```python
from build123d import *

# Parameters (mm, degrees)
SKETCH013_R     = 3.96875
PAD009_DEPTH    = 164
SKETCH014_R     = 7.5
PAD010_DEPTH    = 10
SKETCH015_R     = 7.5
POCKET003_DEPTH = 8
SKETCH016_R     = 7.5
SKETCH016_R_2   = 3.96875
POCKET004_DEPTH = 2
SKETCH017_R     = 7.5
PAD011_DEPTH    = 10
SKETCH018_R     = 7.5
POCKET005_DEPTH = 8
SKETCH019_R     = 7.5
SKETCH019_R_2   = 3.96875
POCKET006_DEPTH = 2


with BuildPart() as part:
    # Sketch013 → Pad009 (new body)
    with BuildSketch(Plane(origin=(500, 82, 56), x_dir=(1, 0, 0), z_dir=(0, -1, 0))):
        Circle(SKETCH013_R)
    extrude(amount=PAD009_DEPTH)

    # Sketch014 → Pad010 (new body)
    with BuildSketch(Plane(origin=(500, 82, 56), x_dir=(1, 0, 0), z_dir=(0, 1, 0))):
        Circle(SKETCH014_R)
    extrude(amount=-PAD010_DEPTH)

    # Sketch015 → Pocket003 (cut)
    with BuildSketch(Plane(origin=(500, 82, 56), x_dir=(1, 0, 0), z_dir=(0, 1, 0))):
        Circle(SKETCH015_R)
        Polygon((0, 5), (-4.330127, 2.5), (-4.330127, -2.5), (0, -5), (4.330127, -2.5), (4.330127, 2.5), align=None, mode=Mode.SUBTRACT)
    extrude(amount=-POCKET003_DEPTH, mode=Mode.SUBTRACT)

    # Sketch016 → Pocket004 (cut)
    with BuildSketch(Plane(origin=(500, 82, 56), x_dir=(1, 0, 0), z_dir=(0, 1, 0))):
        Circle(SKETCH016_R)
        Circle(SKETCH016_R_2, mode=Mode.SUBTRACT)
    extrude(amount=-POCKET004_DEPTH, mode=Mode.SUBTRACT)

    # Sketch017 → Pad011 (new body)
    with BuildSketch(Plane(origin=(500, -82, 56), x_dir=(1, 0, 0), z_dir=(0, -1, 0))):
        Circle(SKETCH017_R)
    extrude(amount=-PAD011_DEPTH)

    # Sketch018 → Pocket005 (cut)
    with BuildSketch(Plane(origin=(500, -82, 56), x_dir=(1, 0, 0), z_dir=(0, -1, 0))):
        Circle(SKETCH018_R)
        Polygon((0, 5), (-4.330127, 2.5), (-4.330127, -2.5), (0, -5), (4.330127, -2.5), (4.330127, 2.5), align=None, mode=Mode.SUBTRACT)
    extrude(amount=-POCKET005_DEPTH, mode=Mode.SUBTRACT)

    # Sketch019 → Pocket006 (cut)
    with BuildSketch(Plane(origin=(500, -82, 56), x_dir=(1, 0, 0), z_dir=(0, -1, 0))):
        Circle(SKETCH019_R)
        Circle(SKETCH019_R_2, mode=Mode.SUBTRACT)
    extrude(amount=-POCKET006_DEPTH, mode=Mode.SUBTRACT)


with BuildPart() as part_1:
    # Clone020 placement: moved
    add(part.part.moved(Location((-951.5, 0, -84))))


solid = part_1.part
```
Model file for the job. Use its own axes, mm. A direction names the side the tool comes from. Coordinates: 2 decimals unless noted, no trailing zeros. Order: outer loops, then holes, each group sorted by start corner. A loop starts at its lowest first (then second) coordinate and runs counter-clockwise, first axis right, second up. Notation, with made-up numbers: (89.25, -33.75) -> (123.25, -33.75) arc R24 cw to (123.25, -4.75) -> close; hole circle Ø8 at (-40, -26.5). An arc over 180 degrees is marked (long way). Return JSON: item names as keys, results as strings.
Item 1: Wall check: line 1 along Y through (x, z) = (-453.5, -33.5); line 2 along Y through (x, z) = (-447.5, -28.5); line 3 along X through (y, z) = (-49, -25.5). Give the ranges that are in metal, low to high. Write a range as from..to.
Model answer:
{"line 1": "y = -74..-72, 72..74", "line 2": "y = -80..-72, 72..80", "line 3": "x = -454.58..-448.42"}
Item 2: Slice it at C-C (y = 12). Write the cut outline in (x, z), then the cut area to 3 significant figures.
Model answer:
{"outline": "circle Ø7.94 at (-451.5, -28)", "area": "49.5 mm²"}
Item 3: Slice it at A-A (z = -28). Write the cut outline in (x, y).
Model answer:
{"outline": "(-459, -74) -> (-455.83, -74) -> (-455.83, -80) -> (-455.47, -80) -> (-455.47, -82) -> (-447.53, -82) -> (-447.53, -80) -> (-447.17, -80) -> (-447.17, -74) -> (-444, -74) -> (-444, -72) -> (-447.53, -72) -> (-447.53, 72) -> (-444, 72) -> (-444, 74) -> (-447.17, 74) -> (-447.17, 80) -> (-447.53, 80) -> (-447.53, 82) -> (-455.47, 82) -> (-455.47, 80) -> (-455.83, 80) -> (-455.83, 74) -> (-459, 74) -> (-459, 72) -> (-455.47, 72) -> (-455.47, -72) -> (-459, -72) -> close"}
Item 4: Pin check, flat tips, straight feed: P1, Ø1.5, axis at y = -35, z = -31, coming from the -X side; P2, Ø2.5, axis at y = 76.5, z = -27.5, coming from the -X side; P3, Ø1.5, axis at y = -75.5, z = -28, coming from the +X side. Stop position of each tip, or through.
Model answer:
{"P1": "stops at x = -454.77", "P2": "stops at x = -455.83", "P3": "stops at x = -447.17"}
Item 5: Slice it at B-B (x = -449.5). Write the cut outline in (y, z), then the cut area to 3 significant figures.
Model answer:
{"outline": "(-82, -31.43) -> (-80, -31.43) -> (-80, -31.85) -> (-74, -31.85) -> (-74, -35.23) -> (-72, -35.23) -> (-72, -31.43) -> (72, -31.43) -> (72, -35.23) -> (74, -35.23) -> (74, -31.85) -> (80, -31.85) -> (80, -31.43) -> (82, -31.43) -> (82, -24.57) -> (80, -24.57) -> (80, -24.15) -> (74, -24.15) -> (74, -20.77) -> (72, -20.77) -> (72, -24.57) -> (-72, -24.57) -> (-72, -20.77) -> (-74, -20.77) -> (-74, -24.15) -> (-80, -24.15) -> (-80, -24.57) -> (-82, -24.57) -> close", "area": "1,160 mm²"}
Item 6: 3-axis set-ups, long thin cutter, end or side, ignore diameter. For faces 1 (the face through (-449.3, -77.04, -24.27)), 2 (the face through (-455.465, 1.008, -27.826)), 3 (the face through (-455.465, 81.014, -28.174)), 4 (the face through (-453.63, -77.04, -24.23)): which of +Z, -Z, +X, -X, +Y, -Y reach the whole face in a straight line?
Model answer:
{"face 1": "+Z, +X, -Y", "face 2": "none", "face 3": "+Y", "face 4": "+Z, -X, -Y"}
Item 7: Mould opens along Y. For faces 5 (the face through (-447.17, 77, -28)), 6 (the face through (-452, -82, -28)), 7 (the face through (-448, 72, -25)) say: pulls with the +Y half, pulls with the -Y half, needs draft (parallel to the pull), parting line crosses it, or undercut.
Model answer:
{"face 5": "needs draft", "face 6": "pulls with the -Y half", "face 7": "undercut"}
